from build123d import *

# Parameters (mm, degrees)
SKETCH022_W     = 87.5
SKETCH022_H     = 89.2
PAD013_DEPTH    = 3
POCKET010_DEPTH = 5
CHAMFER013_SIZE = 2
SKETCH025_W     = 164
SKETCH025_H     = 69.2
PAD015_DEPTH    = 3
FILLET004_R     = 5
SKETCH026_R     = 2.25
POCKET011_DEPTH = 7
CHAMFER014_SIZE = 1
CHAMFER015_SIZE = 0.4


with BuildPart() as part:
    # Sketch022 (on XZ_Plane007 of Origin026) → Pad013 (new body)
    with BuildSketch(Plane.XZ):
        with Locations((43.75, 0)):
            Rectangle(SKETCH022_W, SKETCH022_H)
    extrude(amount=PAD013_DEPTH)

    # Sketch023 (on XZ_Plane007 of Origin026) → Pocket010 (cut)
    with BuildSketch(Plane.XZ):
        with BuildLine():
            ThreePointArc((76.5, 39.8), (78.2, 41.5), (76.5, 43.2))
            Line((76.5, 43.2), (66.5, 43.2))
            ThreePointArc((66.5, 43.2), (64.8, 41.5), (66.5, 39.8))
            Line((76.5, 39.8), (66.5, 39.8))
        make_face()
    pocket010 = extrude(amount=POCKET010_DEPTH, mode=Mode.SUBTRACT)

    # Mirrored008: Pocket010 across XY
    add(pocket010.mirror(Plane.XY), mode=Mode.SUBTRACT)

    # Mirrored009: part across YZ


with BuildPart() as part_1:
    add(part.part)
    add(part.part.mirror(Plane.YZ))

    # Chamfer013
    chamfer013_edges = [part_1.edges().sort_by_distance(p)[0] for p in [
        (-87.5, -1.5, 44.6),
        (-87.5, -1.5, -44.6),
        (87.5, -1.5, 44.6),
        (87.5, -1.5, -44.6),
    ]]
    chamfer(chamfer013_edges, length=CHAMFER013_SIZE)

    # Sketch025 → Pad015 (join)
    with BuildSketch(Plane.XZ.offset(3)):
        Rectangle(SKETCH025_W, SKETCH025_H)
    extrude(amount=PAD015_DEPTH)

    # Fillet004
    fillet004_edges = [part_1.edges().sort_by_distance(p)[0] for p in [
        (82, -4.5, 34.6),
        (82, -4.5, -34.6),
        (-82, -4.5, 34.6),
        (-82, -4.5, -34.6),
    ]]
    fillet(fillet004_edges, radius=FILLET004_R)

    # Sketch026 (on Face34 of Fillet004) → Pocket011 (cut)
    with BuildSketch(Plane.XZ.offset(6)):
        with Locations((-75, 25)):
            Circle(SKETCH026_R)
        with Locations((-25, 25)):
            Circle(SKETCH026_R)
        with Locations((25, 25)):
            Circle(SKETCH026_R)
        with Locations((75, 25)):
            Circle(SKETCH026_R)
        with Locations((75, -25)):
            Circle(SKETCH026_R)
        with Locations((25, -25)):
            Circle(SKETCH026_R)
        with Locations((-25, -25)):
            Circle(SKETCH026_R)
        with Locations((-75, -25)):
            Circle(SKETCH026_R)
    extrude(amount=-POCKET011_DEPTH, mode=Mode.SUBTRACT)

    # Chamfer014
    chamfer014_edges = [part_1.edges().sort_by_distance(p)[0] for p in [
        (0, -6, -34.6),
        (-80.535534, -6, -33.135534),
        (80.535534, -6, -33.135534),
        (-82, -6, 0),
        (82, -6, 0),
        (-80.535534, -6, 33.135534),
        (80.535534, -6, 33.135534),
        (0, -6, 34.6),
        (-77.25, -6, -25),
        (-27.25, -6, -25),
        (-77.25, -6, 25),
        (-27.25, -6, 25),
        (22.75, -6, -25),
        (72.75, -6, -25),
        (22.75, -6, 25),
        (72.75, -6, 25),
    ]]
    chamfer(chamfer014_edges, length=CHAMFER014_SIZE)

    # Chamfer015
    chamfer015_edges = [part_1.edges().sort_by_distance(p)[0] for p in [
        (0, 0, -44.6),
        (86.5, 0, -43.6),
        (-86.5, 0, -43.6),
        (87.5, 0, 0),
        (-87.5, 0, 0),
        (86.5, 0, 43.6),
        (-86.5, 0, 43.6),
        (0, 0, 44.6),
        (-78.2, 0, -41.5),
        (-71.5, 0, -39.8),
        (-71.5, 0, -43.2),
        (-64.8, 0, -41.5),
        (-77.25, 0, -25),
        (-27.25, 0, -25),
        (-77.25, 0, 25),
        (-71.5, 0, 39.8),
        (-78.2, 0, 41.5),
        (-64.8, 0, 41.5),
        (-71.5, 0, 43.2),
        (-27.25, 0, 25),
        (22.75, 0, -25),
        (78.2, 0, -41.5),
        (71.5, 0, -39.8),
        (71.5, 0, -43.2),
        (64.8, 0, -41.5),
        (72.75, 0, -25),
        (22.75, 0, 25),
        (72.75, 0, 25),
        (71.5, 0, 39.8),
        (78.2, 0, 41.5),
        (64.8, 0, 41.5),
        (71.5, 0, 43.2),
    ]]
    chamfer(chamfer015_edges, length=CHAMFER015_SIZE)


solid = part_1.part
Check sheet for the modelled part. Datum: model origin and axes. Units: mm. A direction names the side the tool comes from. Round coordinates to 2 decimals unless told otherwise and drop trailing zeros. Loops run counter-clockwise (first coordinate to the right, second up) from the corner with the lowest first, then second, coordinate; pieces in that order, holes last.
1. Gauge pin test, flat ends, axial feed: pin 1 Ø5 at (x, z) = (-25, 25) entering from -Y; pin 2 Ø0.6 at (x, y) = (-8, -3.5) entering from +Z; pin 3 Ø2 at (y, z) = (-4.5, 1.5) entering from +X. Record the tip position at first contact, or that the pin passes through.
2. Sectioned sample at A-A on x = 31. Record the boundary of the cut face in (y, z).
3. Sectioned sample at C-C on z = -10.5. Record the boundary of the cut face in (x, y).
4. Set-up check for faces 1 (the cylindrical face through (-80.57, -4.01, -33.1)), 2 (the cylindrical face through (80.5, -4.01, 33.17)), 3 (the cylindrical face through (76.038, -2.732, -26.996)): record each of +Z, -Z, +X, -X, +Y, -Y from which the full face is reachable in a straight line by a thin tool's end or side.
5. Scan lines: probe 1 along X at (y, z) = (-1, 41.5); probe 2 along Z at (x, y) = (-25, -1.6); probe 3 along Z at (x, y) = (75, -2.8). Record each from-to range of solid material in increasing order.
6. Mould release check, pull along X, two halves, no side actions. Record for faces 4 (the conical face through (-80.05, -5.73, -32.59)), 5 (the cylindrical face through (80.57, -4.01, -33.1)), 6 (the cylindrical face through (-23.962, -2.732, 23.004)): released by +X, released by -X, zero draft, split by the parting line, or undercut.
7. Sectioned sample at B-B on y = -4. Give the number of separate pieces and of enclosed holes in the cut face, and give its area (3 significant figures).
Recorded:
1. pin 1: stops at y = -5.25
1. pin 2: stops at z = 34.6
1. pin 3: stops at x = 82
2. outline: (-6, -33.6) - (-5, -34.6) - (-3, -34.6) - (-3, -44.6) - (-0.4, -44.6) - (0, -44.2) - (0, 44.2) - (-0.4, 44.6) - (-3, 44.6) - (-3, 34.6) - (-5, 34.6) - (-6, 33.6) - close
3. outline: (-87.5, -3) - (-82, -3) - (-82, -5) - (-81, -6) - (81, -6) - (82, -5) - (82, -3) - (87.5, -3) - (87.5, -0.4) - (87.1, 0) - (-87.1, 0) - (-87.5, -0.4) - close
4. face 1: -Z, -X, -Y
4. face 2: +Z, +X, -Y
4. face 3: +Y, -Y
5. probe 1: x = -87.5 to -78.2, -64.8 to 64.8, 78.2 to 87.5
5. probe 2: z = -44.6 to -27.25, -22.75 to 22.75, 27.25 to 44.6
5. probe 3: z = -44.6 to -43.2, -39.8 to -27.25, -22.75 to 22.75, 27.25 to 39.8, 43.2 to 44.6
6. face 4: released by -X
6. face 5: released by +X
6. face 6: undercut
7. separate pieces: 1
7. enclosed holes: 8
7. area: 11,200 mm2
